from build123d import *

# Parameters (mm, degrees)
F1_DEPTH = 25.4


with BuildPart() as f1:
    # F0 (on Right) → F1 (new body)
    with BuildSketch(Plane.YZ):
        with BuildLine():
            ThreePointArc((77.7355076163, 35.4636907578), (76.6675961502, 47.7624663657), (73.4958271318, 59.6931074906))
            Line((73.4958271318, 59.6931074906), (69.2378436874, 1.6926861527))
            ThreePointArc((69.2378436874, 1.6926861527), (75.5784886533, 18.0518338473), (77.7355076163, 35.4636907578))
        make_face()
        with BuildLine():
            Line((69.2378436874, 1.6926861527), (73.4958271318, 59.6931074906))
            ThreePointArc((73.4958271318, 59.6931074906), (68.3879297776, 70.7709703077), (61.4677361542, 80.8168938687))
            add(Edge.make_bspline(
                [(46.7271482261, 23.3890579279), (57.3671713501, 38.6358972227), (67.4277924366, 61.0196278452), (62.6176115866, 78.1431138882), (61.4677361542, 80.8168938687)],
                knots=[0.2275291842, 0.2275291842, 0.2275291842, 0.2275291842, 0.3610428006, 0.3876214238, 0.3876214238, 0.3876214238, 0.3876214238], degree=3))
            ThreePointArc((46.7271482261, 23.3890579279), (58.8331802448, 12.9122292433), (68.2986060932, 0))
            ThreePointArc((68.2986060932, 0), (68.7739653696, 0.8431577995), (69.2378436874, 1.6926861527))
        make_face()
        with BuildLine():
            Line((69.0189883561, -1.2884671556), (69.2378436874, 1.6926861527))
            ThreePointArc((69.2378436874, 1.6926861527), (68.7739653696, 0.8431577995), (68.2986060932, 0))
            ThreePointArc((68.2986060932, 0), (68.6621292842, -0.6423706226), (69.0189883561, -1.2884671556))
        make_face()
        with BuildLine():
            add(Edge.make_bspline(
                [(46.7271482261, 23.3890579279), (57.3671713501, 38.6358972227), (67.4277924366, 61.0196278452), (62.6176115866, 78.1431138882), (61.4677361542, 80.8168938687)],
                knots=[0.2275291842, 0.2275291842, 0.2275291842, 0.2275291842, 0.3610428006, 0.3876214238, 0.3876214238, 0.3876214238, 0.3876214238], degree=3))
            ThreePointArc((61.4677361542, 80.8168938687), (42.6716941747, 96.9001796523), (19.5137307938, 105.5991455529))
            add(Edge.make_bspline(
                [(19.5137307938, 105.5991455529), (15.2484459589, 105.6418292249), (-17.4670589129, 101.9834872227), (-51.4356414133, 56.0713753865), (-36.7498246069, 29.4728703431), (-32.4913798704, 24.3725458831)],
                knots=[0.5361274609, 0.5361274609, 0.5361274609, 0.5361274609, 0.5710508717, 0.8014313121, 0.8647451677, 0.8647451677, 0.8647451677, 0.8647451677], degree=3))
            ThreePointArc((-32.4913798704, 24.3725458831), (-6.4015352071, 34.736385461), (21.6668981331, 34.2341751698))
            ThreePointArc((21.6668981331, 34.2341751698), (34.7206440257, 30.0215683701), (46.7271482261, 23.3890579279))
        make_face()
        with BuildLine():
            ThreePointArc((19.5137307938, 105.5991455529), (42.6716941747, 96.9001796523), (61.4677361542, 80.8168938687))
            add(Edge.make_bspline(
                [(61.4677361542, 80.8168938687), (55.0428945656, 95.7564363048), (37.6511501332, 105.4176402871), (19.5137307938, 105.5991455529)],
                knots=[0.3876214238, 0.3876214238, 0.3876214238, 0.3876214238, 0.5361274609, 0.5361274609, 0.5361274609, 0.5361274609], degree=3))
        make_face()
        with BuildLine():
            ThreePointArc((77.7355076163, -35.4636907578), (75.5220462625, -17.829040093), (69.0189883561, -1.2884671556))
            Line((69.0189883561, -1.2884671556), (64.0810679537, -68.550697648))
            add(Edge.make_bspline(
                [(64.0810679537, -68.550697648), (64.055573163, -69.8265995508), (63.9650070893, -71.0818079643), (63.8049086741, -72.3124207221)],
                knots=[0.3500957655, 0.3500957655, 0.3500957655, 0.3500957655, 0.3610428006, 0.3610428006, 0.3610428006, 0.3610428006], degree=3))
            add(Edge.make_bspline(
                [(63.8049086741, -72.3124207221), (63.4162011029, -75.3002610177), (62.6176115866, -78.1431138882), (61.4677361542, -80.8168938687)],
                knots=[0.3610428006, 0.3610428006, 0.3610428006, 0.3610428006, 0.3876214238, 0.3876214238, 0.3876214238, 0.3876214238], degree=3))
            ThreePointArc((61.4677361542, -80.8168938687), (73.5455465545, -59.5549413519), (77.7355076163, -35.4636907578))
        make_face()
        with BuildLine():
            Line((64.0810679537, -68.550697648), (69.0189883561, -1.2884671556))
            ThreePointArc((69.0189883561, -1.2884671556), (68.6621292842, -0.6423706226), (68.2986060932, 0))
            ThreePointArc((68.2986060932, 0), (58.8331802447, -12.9122292433), (46.7271482261, -23.3890579279))
            add(Edge.make_bspline(
                [(46.7271482261, -23.3890579279), (56.4947756325, -37.3857798919), (64.3665159576, -54.2652831945), (64.0810679537, -68.550697648)],
                knots=[0.2275291842, 0.2275291842, 0.2275291842, 0.2275291842, 0.3500957655, 0.3500957655, 0.3500957655, 0.3500957655], degree=3))
        make_face()
        with BuildLine():
            add(Edge.make_bspline(
                [(19.5137307938, 105.5991455529), (15.2484459589, 105.6418292249), (-17.4670589129, 101.9834872227), (-51.4356414133, 56.0713753865), (-36.7498246069, 29.4728703431), (-32.4913798704, 24.3725458831)],
                knots=[0.5361274609, 0.5361274609, 0.5361274609, 0.5361274609, 0.5710508717, 0.8014313121, 0.8647451677, 0.8647451677, 0.8647451677, 0.8647451677], degree=3))
            ThreePointArc((19.5137307938, 105.5991455529), (-51.7805921013, 76.7996475885), (-55.5363464012, 0))
            ThreePointArc((-55.5363464012, 0), (-45.4663442086, 13.5596369664), (-32.4913798704, 24.3725458831))
        make_face()
        with BuildLine():
            Line((63.8049086741, -72.3124207222), (64.0810679537, -68.550697648))
            add(Edge.make_bspline(
                [(46.7271482261, -23.3890579279), (56.4947756325, -37.3857798919), (64.3665159576, -54.2652831945), (64.0810679537, -68.550697648)],
                knots=[0.2275291842, 0.2275291842, 0.2275291842, 0.2275291842, 0.3500957655, 0.3500957655, 0.3500957655, 0.3500957655], degree=3))
            ThreePointArc((46.7271482261, -23.3890579279), (33.6000701349, -30.4952094493), (19.2818065466, -34.7147943189))
            ThreePointArc((19.2818065466, -34.7147943189), (-7.5965149208, -34.5082512887), (-32.4913798704, -24.3725458831))
            add(Edge.make_bspline(
                [(19.5137307938, -105.5991455529), (15.2484459589, -105.6418292249), (-17.4670589129, -101.9834872227), (-51.4356414133, -56.0713753865), (-36.7498246069, -29.4728703431), (-32.4913798704, -24.3725458831)],
                knots=[0.5361274609, 0.5361274609, 0.5361274609, 0.5361274609, 0.5710508717, 0.8014313121, 0.8647451677, 0.8647451677, 0.8647451677, 0.8647451677], degree=3))
            ThreePointArc((19.5137307938, -105.5991455529), (42.6716941747, -96.9001796523), (61.4677361542, -80.8168938687))
            add(Edge.make_bspline(
                [(63.8049086741, -72.3124207221), (63.4162011029, -75.3002610177), (62.6176115866, -78.1431138882), (61.4677361542, -80.8168938687)],
                knots=[0.3610428006, 0.3610428006, 0.3610428006, 0.3610428006, 0.3876214238, 0.3876214238, 0.3876214238, 0.3876214238], degree=3))
        make_face()
        with BuildLine():
            ThreePointArc((-32.4913798704, 24.3725458831), (-45.4663442086, 13.5596369664), (-55.5363464012, 0))
            ThreePointArc((-55.5363464012, 0), (-45.4663442086, -13.5596369664), (-32.4913798704, -24.3725458831))
            add(Edge.make_bspline(
                [(-32.4913798704, -24.3725458831), (-23.3942363951, -13.4769287613), (-9.3112886841, -5.4733246177), (0, 0)],
                knots=[0.8647451677, 0.8647451677, 0.8647451677, 0.8647451677, 1, 1, 1, 1], degree=3))
            add(Edge.make_bspline(
                [(-32.4913798704, 24.3725458831), (-23.3942363951, 13.4769287613), (-9.3112886841, 5.4733246177), (0, 0)],
                knots=[0.8647451677, 0.8647451677, 0.8647451677, 0.8647451677, 1, 1, 1, 1], degree=3))
        make_face()
        with BuildLine():
            ThreePointArc((-32.4913798704, -24.3725458831), (-45.4663442086, -13.5596369664), (-55.5363464012, 0))
            ThreePointArc((-55.5363464012, 0), (-51.7805921013, -76.7996475885), (19.5137307938, -105.5991455529))
            add(Edge.make_bspline(
                [(19.5137307938, -105.5991455529), (15.2484459589, -105.6418292249), (-17.4670589129, -101.9834872227), (-51.4356414133, -56.0713753865), (-36.7498246069, -29.4728703431), (-32.4913798704, -24.3725458831)],
                knots=[0.5361274609, 0.5361274609, 0.5361274609, 0.5361274609, 0.5710508717, 0.8014313121, 0.8647451677, 0.8647451677, 0.8647451677, 0.8647451677], degree=3))
        make_face()
        with BuildLine():
            add(Edge.make_bspline(
                [(61.4677361542, -80.8168938687), (55.0428945656, -95.7564363048), (37.6511501332, -105.4176402871), (19.5137307938, -105.5991455529)],
                knots=[0.3876214238, 0.3876214238, 0.3876214238, 0.3876214238, 0.5361274609, 0.5361274609, 0.5361274609, 0.5361274609], degree=3))
            ThreePointArc((61.4677361542, -80.8168938687), (42.6716941747, -96.9001796523), (19.5137307938, -105.5991455529))
        make_face()
    extrude(amount=F1_DEPTH)


solid = f1.part
Part model, mm, in its own coordinate system. Coordinates: 2 decimals unless noted, no trailing zeros. Loops run counter-clockwise (first coordinate to the right, second up) from the corner with the lowest first, then second, coordinate; pieces in that order, holes last. Notation, with made-up numbers: M 29,12 L 62,12 A27 cw 62,31 Z; hole C -12.5,45.5 d1. An arc over 180 degrees is marked long. Use a Markdown table: item, result. Add a question column.
Q1. Cut at A-A (z = 32). Write the cut outline in (x, y).
Q2. Probe L1, parallel to Z at x = 15.5, y = 4; L2, parallel to Z at x = 18.75, y = -32; L3, parallel to Y at x = 16.75, z = -26.5. List the from-to ranges inside material, lowest first.
Q3. Cut at C-C (x = 2.5). Give the number of separate pieces and of enclosed holes in the cut face, and give its area (3 significant figures).
Q4. Cut at B-B (y = -43). Write the cut outline in (x, z), and give its area (3 significant figures).
Q5. Pin check, flat tips, straight feed: P1, Ø6, axis at y = -18.5, z = -41.5, coming from the -X side; P2, Ø4, axis at x = 18, y = 45, coming from the -Z side; P3, Ø10, axis at x = 16.5, y = 19.5, coming from the +Z side; P4, Ø8, axis at x = 20.5, y = 48, coming from the -Z side. Stop position of each tip, or through.
Q6. Cut at D-D (z = 56). Write the cut outline in (x, y).
Q7. Mould opens along Z. For faces 1 (the flat face through (25.4, -10, 1)), 2 (the cylindrical face through (12.52, -52.43, -75.87)) say: +Z half, -Z half, draft (parallel to the pull), parting line (faces both ways), or undercut.
Worked out:
| question | item | result |
|---|---|---|
| 1 | outline | M 0,-64.89 L 25.4,-64.89 L 25.4,-16.86 L 0,-16.86 Z; M 0,29.62 L 25.4,29.62 L 25.4,77.65 L 0,77.65 Z |
| 2 | L1 | z = -106.78 to -35.85, 35.85 to 106.78 |
| 2 | L2 | z = -95.62 to -24.69, -23.79 to 23.79, 24.69 to 95.62 |
| 2 | L3 | y = -64.41 to -29, 41.76 to 77.17 |
| 3 | separate pieces | 1 |
| 3 | enclosed holes | 2 |
| 3 | area | 20,900 mm2 |
| 4 | outline | M 0,-86.97 L 25.4,-86.97 L 25.4,86.97 L 0,86.97 Z |
| 4 | area | 4,420 mm2 |
| 5 | P1 | stops at x = 0 |
| 5 | P2 | stops at z = -99.78 |
| 5 | P3 | stops at z = 106.35 |
| 5 | P4 | stops at z = -99.24 |
| 6 | outline | M 0,-61.95 L 25.4,-61.95 L 25.4,74.72 L 0,74.72 Z |
| 7 | face 1 | draft |
| 7 | face 2 | undercut |
